from build123d import *

# Parameters (mm, degrees)
SKETCH1_R               = 6.477
BOSS_EXTRUDE1_DEPTH     = 10.795
CUT_EXTRUDE3_DEPTH      = 64.211808035
CUT_EXTRUDE3_DEPTH_BACK = 64.211808035
SKETCH8_R               = 1.55
SKETCH9_R               = 3.81
CUT_EXTRUDE4_DEPTH      = 64.211808035
CUT_EXTRUDE5_DEPTH      = 64.211808035
FILLET1_R               = 1.016
SKETCH13_W              = 22.225
SKETCH13_H              = 9.4
CUT_EXTRUDE6_DEPTH      = 63.22676012
FILLET7_R               = 2.54
CHAMFER2_SIZE           = 0.508


with BuildPart() as part:
    # Sketch1 → Boss-Extrude1 (new body)
    with BuildSketch(Plane(origin=(0, 0, 0), x_dir=(1, 0, 0), z_dir=(0, 1, 0))):
        with BuildLine():
            Line((1.744418558, 10.653122964), (38.1, 4.7))
            Line((38.1, 4.7), (60.325, 4.7))
            Line((60.325, 4.7), (60.325, 1.525))
            Line((60.325, 1.525), (15.875, 1.525))
            Line((15.875, 1.525), (15.875, -1.525))
            Line((15.875, -1.525), (60.325, -1.525))
            Line((60.325, -1.525), (60.325, -4.7))
            Line((60.325, -4.7), (38.1, -4.7))
            Line((38.1, -4.7), (1.744418558, -10.653122964))
            ThreePointArc((1.744418558, -10.653122964), (-10.795, 0), (1.744418558, 10.653122964))
        make_face()
        with Locations(Location((0, 0, 0), (0, 0, 270))):
            Circle(SKETCH1_R, mode=Mode.SUBTRACT)
    extrude(amount=BOSS_EXTRUDE1_DEPTH)

    # Sketch8 → Cut-Extrude3 (cut, two sides: drawn at the far end of the back side and taken through both)
    with BuildSketch(Plane.XY.offset(4.7).offset(-CUT_EXTRUDE3_DEPTH_BACK)):
        with Locations((26.9875, 5.3975)):
            Circle(SKETCH8_R)
        with Locations((49.2125, 5.3975)):
            Circle(SKETCH8_R)
    extrude(amount=CUT_EXTRUDE3_DEPTH + CUT_EXTRUDE3_DEPTH_BACK, mode=Mode.SUBTRACT)

    # Sketch9 → Cut-Extrude4 (cut, through all)
    with BuildSketch(Plane.XY.offset(4.7)):
        with Locations((26.9875, 5.3975)):
            Circle(SKETCH9_R)
    extrude(amount=CUT_EXTRUDE4_DEPTH, mode=Mode.SUBTRACT)

    # Sketch10 → Cut-Extrude5 (cut, through all)
    with BuildSketch(Plane(origin=(0, 0, -4.7), x_dir=(-1, 0, 0), z_dir=(0, 0, -1))):
        Polygon((-24.13, 3.747721606), (-24.13, 7.047278394), (-26.9875, 8.697056788), (-29.845, 7.047278394), (-29.845, 3.747721606), (-26.9875, 2.097943212), align=None)
    extrude(amount=CUT_EXTRUDE5_DEPTH, mode=Mode.SUBTRACT)

    # Fillet1
    fillet1_edges = [part.edges().sort_by_distance(p)[0] for p in [
        (15.875, 5.3975, -1.525),
        (15.875, 5.3975, 1.525),
    ]]
    fillet(fillet1_edges, radius=FILLET1_R)

    # Sketch13 → Cut-Extrude6 (cut, through all)
    with BuildSketch(Plane.XZ):
        with Locations((49.2125, 0)):
            Rectangle(SKETCH13_W, SKETCH13_H)
    extrude(amount=-CUT_EXTRUDE6_DEPTH, mode=Mode.SUBTRACT)

    # Fillet7
    fillet7_edges = [part.edges().sort_by_distance(p)[0] for p in [
        (38.1, 5.3975, -4.7),
        (38.1, 5.3975, 4.7),
    ]]
    fillet(fillet7_edges, radius=FILLET7_R)

    # Chamfer2
    chamfer2_edges = [part.edges().sort_by_distance(p)[0] for p in [
        (0, 0, -6.477),
        (0, 10.795, -6.477),
    ]]
    chamfer(chamfer2_edges, length=CHAMFER2_SIZE)


solid = part.part
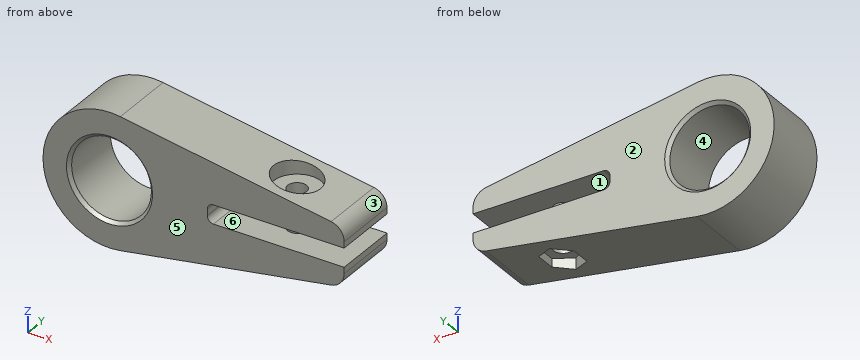
Can you work these out from the model? Positions are in its coordinate system, mm. Face numbers are marked on the shaded views. A direction names the side the tool comes from. Give positions to 0.01 mm unless a question says otherwise; leave off trailing zeros. Order: outer loops, then holes, each group sorted by start corner. A loop starts at its lowest first (then second) coordinate and runs counter-clockwise, first axis right, second up. Notation, with made-up numbers: M 56.25,-26 L 104.25,-26 A20 ccw 104.25,-16 Z; hole C 67,-40 d6. An arc over 180 degrees is marked long. Use one line per item in the form item = value. Start each with the question number.
Item 1: If we section it at C-C (y = 4.75): State how many separate pieces and enclosed holes the cut face has, then the cut area to 3 significant figures.
Item 2: We'd pull the mould along Z, two halves only. Please class the marked faces 3, 4, 5 and 6: +Z half, -Z half, draft (parallel to the pull), parting line (faces both ways), or undercut.
Item 3: For the marked faces 1 and 2, which set-ups out of +Z, -Z, +X, -X, +Y, -Y let a thin tool reach every point of the face, with its end or its side?
Item 4: If I drill on line 1 along X through (y, z) = (4.75, 0) (3 decimals); line 2 along Z through (x, y) = (1.5, 1.5); line 3 along X through (y, z) = (2, -1.25), over which ranges is the centre line in solid material (lowest first)?
Item 5: If we section it at B-B (x = 33): Write out the boundary of the cut face in (y, z) (3 decimals).
Item 6: If we section it at A-A (z = 0): Write out the boundary of the cut face in (x, y) (3 decimals), then the cut area to 3 significant figures.
Item 7: Will these pins go through, and if not, where does the flat tip stop? pin 1 Ø2.5 at (x, y) = (27, 4) entering from +Z; pin 2 Ø4 at (x, y) = (26.99, 5.4) entering from -Z; pin 3 Ø6 at (x, y) = (-5.5, 3.5) entering from -Z; pin 4 Ø11.5 at (x, z) = (0, 0) entering from -Y.
Outcome:
q1.separate_pieces = 3
q1.enclosed_holes = 1
q1.area = 536 mm2
q2.face_3 = +Z half
q2.face_4 = undercut
q2.face_5 = draft
q2.face_6 = undercut
q3.face_1 = +X, +Y, -Y
q3.face_2 = +Z, -Z, +X, -X, +Y
q4.line_1 = -10.795 to -6.477, 6.477 to 15.875
q4.line_2 = -10.69 to -6.3, 6.3 to 10.69
q4.line_3 = -10.72 to -6.36, 6.36 to 16.2
q5.outline = M 0,-5.535 L 10.795,-5.535 L 10.795,-1.525 L 0,-1.525 Z; M 0,1.525 L 10.795,1.525 L 10.795,5.535 L 0,5.535 Z
q6.outline = M -10.795,0 L -6.985,0 L -6.477,0.508 L -6.477,10.287 L -6.985,10.795 L -10.795,10.795 Z; M 6.477,0.508 L 6.985,0 L 15.875,0 L 15.875,10.795 L 6.985,10.795 L 6.477,10.287 Z
q6.area = 148 mm2
q7.pin_1 = 4.7
q7.pin_2 = -4.7
q7.pin_3 = -10.5
q7.pin_4 = through
